```python
from build123d import *

# Parameters (mm, degrees)
F0_W      = 27
F0_H      = 15.9
F0_W_2    = 15.9
F0_H_2    = 27
F0_W_3    = 3
F0_H_3    = 3
F1_DEPTH  = 21.9
F2_DEPTH  = 51.8
F3_R      = 7.95
F6_DEPTH  = 30
F7_DEPTH  = 30
F4_R      = 7.9
F8_DEPTH  = 30
F10_DEPTH = 51.9
F11_R     = 1.5


with BuildPart() as f1:
    # F0 (on Front) → F1 (new body)
    with BuildSketch(Plane.XZ):
        with BuildLine():
            Line((-34.3576915575, 15.9), (-42.3076915575, 15.9))
            Line((-42.3076915575, 15.9), (-42.3076915575, 7.9499999931))
            ThreePointArc((-42.3076915575, 7.9499999931), (-39.9791904704, 13.571498908), (-34.3576915575, 15.9))
        make_face()
        with BuildLine():
            ThreePointArc((-34.3576915575, 15.9), (-39.9791904704, 13.571498908), (-42.3076915575, 7.9499999931))
            ThreePointArc((-42.3076915575, 7.9499999931), (-39.9791904655, 2.3285010871), (-34.3576915575, 0))
            ThreePointArc((-34.3576915575, 0), (-28.7361926471, 2.3285010896), (-26.4076915575, 7.95))
            ThreePointArc((-26.4076915575, 7.95), (-28.7361926471, 13.5714989104), (-34.3576915575, 15.9))
        make_face()
        Polygon((-42.3076915575, 18.9), (-42.3076915575, 45.9), (-26.4076915575, 45.9), (-26.4076915575, 18.9), (-23.4076915575, 18.9), (-23.4076915575, 48.9), (-45.3076915575, 48.9), (-45.3076915575, 18.9), align=None)
        with Locations((-9.9076915575, 7.95)):
            Rectangle(F0_W, F0_H)
        with Locations((-34.3576915575, 32.4)):
            Rectangle(F0_W_2, F0_H_2)
        with BuildLine():
            ThreePointArc((-34.3576915575, 0), (-39.9791904655, 2.3285010871), (-42.3076915575, 7.9499999931))
            Line((-42.3076915575, 7.9499999931), (-42.3076915575, 0))
            Line((-42.3076915575, 0), (-34.3576915575, 0))
        make_face()
        with BuildLine():
            Line((-26.4076915575, 0), (-26.4076915575, 7.95))
            ThreePointArc((-26.4076915575, 7.95), (-28.7361926471, 2.3285010896), (-34.3576915575, 0))
            Line((-34.3576915575, 0), (-26.4076915575, 0))
        make_face()
        with BuildLine():
            Line((-26.4076915575, 7.95), (-26.4076915575, 15.9))
            Line((-26.4076915575, 15.9), (-34.3576915575, 15.9))
            ThreePointArc((-34.3576915575, 15.9), (-28.7361926471, 13.5714989104), (-26.4076915575, 7.95))
        make_face()
        Polygon((6.5923084425, 18.9), (-23.4076915575, 18.9), (-23.4076915575, 15.9), (3.5923084425, 15.9), (3.5923084425, 0), (-23.4076915575, 0), (-23.4076915575, -3), (6.5923084425, -3), align=None)
        Polygon((-26.4076915575, 18.9), (-42.3076915575, 18.9), (-42.3076915575, 15.9), (-34.3576915575, 15.9), (-26.4076915575, 15.9), align=None)
        Polygon((-23.4076915575, 15.9), (-26.4076915575, 15.9), (-26.4076915575, 7.95), (-26.4076915575, 0), (-23.4076915575, 0), align=None)
        Polygon((-42.3076915575, 15.9), (-42.3076915575, 18.9), (-45.3076915575, 18.9), (-45.3076915575, -3), (-23.4076915575, -3), (-23.4076915575, 0), (-26.4076915575, 0), (-34.3576915575, 0), (-42.3076915575, 0), (-42.3076915575, 7.9499999931), align=None)
        with Locations((-24.9076915575, 17.4)):
            Rectangle(F0_W_3, F0_H_3)
    extrude(amount=F1_DEPTH)

    # F0 (on Front) → F2 (join)
    with BuildSketch(Plane.XZ):
        Polygon((-42.3076915575, 15.9), (-42.3076915575, 18.9), (-45.3076915575, 18.9), (-45.3076915575, -3), (-23.4076915575, -3), (-23.4076915575, 0), (-26.4076915575, 0), (-34.3576915575, 0), (-42.3076915575, 0), (-42.3076915575, 7.9499999931), align=None)
        with BuildLine():
            ThreePointArc((-34.3576915575, 15.9), (-39.9791904704, 13.571498908), (-42.3076915575, 7.9499999931))
            ThreePointArc((-42.3076915575, 7.9499999931), (-39.9791904655, 2.3285010871), (-34.3576915575, 0))
            ThreePointArc((-34.3576915575, 0), (-28.7361926471, 2.3285010896), (-26.4076915575, 7.95))
            ThreePointArc((-26.4076915575, 7.95), (-28.7361926471, 13.5714989104), (-34.3576915575, 15.9))
        make_face()
        Polygon((-26.4076915575, 18.9), (-42.3076915575, 18.9), (-42.3076915575, 15.9), (-34.3576915575, 15.9), (-26.4076915575, 15.9), align=None)
        Polygon((-23.4076915575, 15.9), (-26.4076915575, 15.9), (-26.4076915575, 7.95), (-26.4076915575, 0), (-23.4076915575, 0), align=None)
        with Locations((-24.9076915575, 17.4)):
            Rectangle(F0_W_3, F0_H_3)
        with BuildLine():
            Line((-26.4076915575, 7.95), (-26.4076915575, 15.9))
            Line((-26.4076915575, 15.9), (-34.3576915575, 15.9))
            ThreePointArc((-34.3576915575, 15.9), (-28.7361926471, 13.5714989104), (-26.4076915575, 7.95))
        make_face()
        with BuildLine():
            Line((-34.3576915575, 15.9), (-42.3076915575, 15.9))
            Line((-42.3076915575, 15.9), (-42.3076915575, 7.9499999931))
            ThreePointArc((-42.3076915575, 7.9499999931), (-39.9791904704, 13.571498908), (-34.3576915575, 15.9))
        make_face()
        with BuildLine():
            ThreePointArc((-34.3576915575, 0), (-39.9791904655, 2.3285010871), (-42.3076915575, 7.9499999931))
            Line((-42.3076915575, 7.9499999931), (-42.3076915575, 0))
            Line((-42.3076915575, 0), (-34.3576915575, 0))
        make_face()
        with BuildLine():
            Line((-26.4076915575, 0), (-26.4076915575, 7.95))
            ThreePointArc((-26.4076915575, 7.95), (-28.7361926471, 2.3285010896), (-34.3576915575, 0))
            Line((-34.3576915575, 0), (-26.4076915575, 0))
        make_face()
    extrude(amount=F2_DEPTH)

    # F3 (on face) → F6 (cut)
    with BuildSketch(Plane.XZ.offset(51.8)):
        with Locations((-34.3576915575, 7.95)):
            Circle(F3_R)
    extrude(amount=-F6_DEPTH, mode=Mode.SUBTRACT)

    # F5 (on face) → F7 (cut)
    with BuildSketch(Plane.YZ.offset(6.5923084425)):
        with BuildLine():
            ThreePointArc((-3, 7.95), (-5.3285010896, 13.5714989104), (-10.95, 15.9))
            ThreePointArc((-10.95, 15.9), (-16.5714989104, 13.5714989104), (-18.9, 7.95))
            ThreePointArc((-18.9, 7.95), (-16.5714989104, 2.3285010896), (-10.95, 0))
            ThreePointArc((-10.95, 0), (-5.3285010896, 2.3285010896), (-3, 7.95))
        make_face()
    extrude(amount=-F7_DEPTH, mode=Mode.SUBTRACT)

    # F4 (on face) → F8 (cut)
    with BuildSketch(Plane.XY.offset(48.9)):
        with Locations((-34.3576915575, -10.9)):
            Circle(F4_R)
    extrude(amount=-F8_DEPTH, mode=Mode.SUBTRACT)

    # F9 (on face) → F10 (join)
    with BuildSketch(Plane(origin=(0, 0, -3), x_dir=(1, 0, 0), z_dir=(0, 0, -1))):
        Polygon((-42.3076915575, 0), (-45.3076915575, 0), (-45.3076915575, -6.3), (-29.0076915575, -6.3), (-29.0076915575, -3.3), (-42.3076915575, -3.3), align=None)
    extrude(amount=-F10_DEPTH)

    # F11
    f11_edges = [f1.edges().sort_by_distance(p)[0] for p in [
        (-35.657692, 3.3, -3),
        (-35.657692, 3.3, 48.9),
    ]]
    fillet(f11_edges, radius=F11_R)


solid = f1.part
```
Input: part model. Units: mm. Frame: model coordinates. A direction names the side the tool comes from. Coordinates: 2 decimals unless noted, no trailing zeros. Loops run counter-clockwise (first coordinate to the right, second up) from the corner with the lowest first, then second, coordinate; pieces in that order, holes last.
Q1. Set-up query: faces 1 (the flat face through (-8, -11, 18.9)), 2 (the cylindrical face through (-42.25, -10.55, 34.11)), 3 (the flat face through (-24, 0, 18)), 4 (the flat face through (-35, -21.9, 34)). Return all of +Z, -Z, +X, -X, +Y, -Y with unobstructed straight access to the full face (end or side cutting, diameter ignored); none if empty.
Results are:
face 1: +Z, +X, +Y, -Y
face 2: +Z
face 3: +Z, -Z, +X
face 4: +Z, +X, -X, -Y
Q2. Section A-A, the plane x = 2.5. Return the cut outline in (y, z).
Results are:
outline: (-21.9, -3) - (0, -3) - (0, 18.9) - (-21.9, 18.9) - close; hole circle Ø15.9 at (-10.95, 7.95)
Q3. Line query: line 1 along Y through (x, z) = (-30, 12); line 2 along X through (y, z) = (-28, 7); line 3 along Z through (x, y) = (-20.5, -10.5). Output: solid intervals per line, ascending.
Results are:
line 1: y = -21.8 to 0, 3.3 to 6.3
line 2: x = -45.31 to -42.25, -26.46 to -23.41
line 3: z = -3 to 0.01, 15.89 to 18.9
Q4. Section C-C, the plane y = -25. Return the cut outline in (x, z).
Results are:
outline: (-45.31, -3) - (-23.41, -3) - (-23.41, 18.9) - (-45.31, 18.9) - close; hole circle Ø15.9 at (-34.36, 7.95)
Q5. Section B-B, the plane z = 26.5. Return the cut outline in (x, y), and give its area (3 significant figures).
Results are:
outline: (-45.31, -21.9) - (-23.41, -21.9) - (-23.41, 0) - (-42.31, 0) - (-42.31, 3.3) - (-29.01, 3.3) - (-29.01, 6.3) - (-45.31, 6.3) - close; hole circle Ø15.8 at (-34.36, -10.9)
area: 342 mm2
Q6. Section D-D, the plane x = -39. Return the cut outline in (y, z), and give its area (3 significant figures).
Results are:
outline: (-51.8, -3) - (0, -3) - (0, 48.9) - (-4.51, 48.9) - (-4.51, 18.9) - (-17.29, 18.9) - (-17.29, 48.9) - (-21.9, 48.9) - (-21.9, 18.9) - (-51.8, 18.9) - (-51.8, 14.4) - (-21.8, 14.4) - (-21.8, 1.5) - (-51.8, 1.5) - close; (3.3, -1.5) arc R1.5 ccw to (4.8, -3) - (6.3, -3) - (6.3, 48.9) - (4.8, 48.9) arc R1.5 ccw to (3.3, 47.4) - close
area: 1,180 mm2
Q7. Contact query for flat-ended pins moving along their axis: pin 1 (2.5 mm diameter, centred on y = 3, z = 20, fed in from +X); pin 2 (6.5 mm diameter, centred on x = -32.5, z = 28.5, fed in from -Y); pin 3 (14.5 mm diameter, centred on x = -34.36, z = 7.95, fed in from -Y); pin 4 (6 mm diameter, centred on x = -21, z = 11.5, fed in from -Y). Output: stop coordinate, or through.
Results are:
pin 1: stops at x = -29.01
pin 2: stops at y = -21.9
pin 3: stops at y = -21.8
pin 4: stops at y = -51.8
Q8. Mould query, pull axis Z, two halves, no side actions, for faces 5 (the cylindrical face through (-27.01, -37.01, 4.91)), 6 (the flat face through (-37, 6.3, 23)), 7 (the flat face through (-25, -23, -3)). Classes: +Z half, -Z half, draft (parallel to the pull), parting line (faces both ways), or undercut.
Results are:
face 5: undercut
face 6: draft
face 7: -Z half
